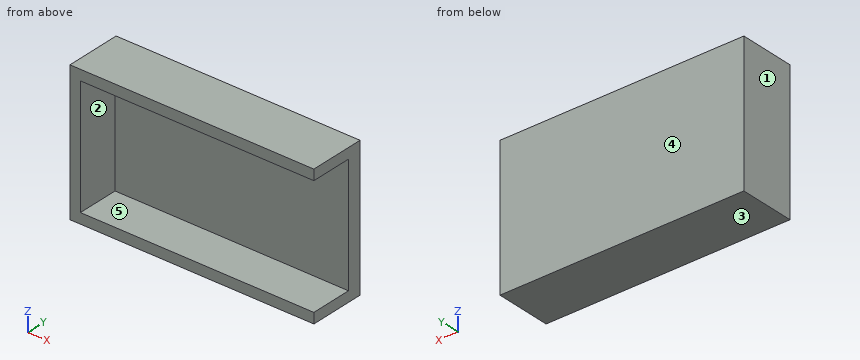
Autodesk Inventor part; units mm, degrees
ref_plane "YZ Plane" through (0, 0, 0) normal (1, 0, 0) x (0, 1, 0)
ref_plane "XZ Plane" through (0, 0, 0) normal (0, 1, 0) x (-1, 0, 0)
ref_plane "XY Plane" through (0, 0, 0) normal (0, 0, 1) x (1, 0, 0)
sketch "Эскиз1" plane through (0, 0, 0) normal (0, 1, 0) x (-1, 0, 0)
  line L0 (-35, 20) -> (35, 20)
  line L1 (35, 20) -> (35, -20)
  line L2 (35, -20) -> (-35, -20)
  line L3 (-35, -20) -> (-35, 20)
  line L4 (-35, 20) -> (35, -20) construction
  line L5 (35, 20) -> (-35, -20) construction
  point P0 (0, 0)
  dimension "d0" = 40
  dimension "d1" = 70
extrude "Выдавливание1" add sketch "Эскиз1" along normal blind 4
sketch "Эскиз2" plane through (0, 0, 0) normal (0, -1, 0) x (1, 0, 0)
  line L0 (-35, 20) -> (35, 20)
  line L1 (35, 20) -> (-35, 20)
  line L2 (-35, 20) -> (-35, 17)
  line L3 (-35, 17) -> (35, 17)
  line L4 (35, 17) -> (35, 20)
  line L5 (35, -20) -> (-35, -20)
  line L6 (35, -20) -> (-35, -20)
  line L7 (-35, -20) -> (-35, -17)
  line L8 (-35, -17) -> (35, -17)
  line L9 (35, -17) -> (35, -20)
  line L10 (-35, -20) -> (-35, 20)
  line L11 (-35, 17) -> (-32, 17)
  line L12 (-32, 17) -> (-32, -17)
  line L13 (-32, -17) -> (-35, -17)
  line L14 (-35, -17) -> (-35, 17)
  point P0 (0, 0)
  dimension "d4" = 3
extrude "Выдавливание2" add sketch "Эскиз2" along normal blind 12
properties part number "Battery box under the board"
Build history of the part. All positions in model axes, mm. Face numbers are marked on the shaded views. A direction names the side the tool comes from. Give positions to 0.01 mm unless a question says otherwise; leave off trailing zeros. Order: outer loops, then holes, each group sorted by start corner. A loop starts at its lowest first (then second) coordinate and runs counter-clockwise, first axis right, second up. Notation, with made-up numbers: M 63.25,33 L 94.25,33 A22 cw 94.25,58 Z; hole C 34.25,-4 d3. An arc over 180 degrees is marked long. Return JSON: item names as keys, results as strings.
Q1. Two-plate mould, pull along Z, no slides. Class the marked faces 3, 4 and 5: pulls with the +Z half, pulls with the -Z half, needs draft (parallel to the pull), parting line crosses it, or undercut.
Answer list:
{"face 3": "pulls with the -Z half", "face 4": "needs draft", "face 5": "undercut"}
Q2. Band-saw the part on A-A (y = -2.25). Give the cut face in (x, z), then the cut area to 3 significant figures.
Answer list:
{"outline": "M -35,-20 L 35,-20 L 35,-17 L -32,-17 L -32,17 L 35,17 L 35,20 L -35,20 Z", "area": "522 mm^2"}
Q3. Wall check: probe 1 along Z at (x, y) = (-15, -4.5); probe 2 along Y at (x, z) = (-18.5, 3); probe 3 along X at (y, z) = (-11, 3). Give the ranges that are in metal, low to high. Write a range as from..to.
Answer list:
{"probe 1": "z = -20..-17, 17..20", "probe 2": "y = 0..4", "probe 3": "x = -35..-32"}
Q4. Flat gauge pins, fed straight in: pin 1 (2 mm diameter, centred on x = -6, z = -7, fed in from -Y); pin 2 (5 mm diameter, centred on y = -7, z = -11.5, fed in from +X); pin 3 (4 mm diameter, centred on x = 1, z = -15.5, fed in from -Y). Where does each tip first touch, or does it go through?
Answer list:
{"pin 1": "stops at y = 0", "pin 2": "stops at x = -32", "pin 3": "stops at y = -12"}
Q5. Band-saw the part on B-B (z = 11.5). Give the cut face in (x, y), then the cut area to 3 significant figures.
Answer list:
{"outline": "M -35,-12 L -32,-12 L -32,0 L 35,0 L 35,4 L -35,4 Z", "area": "316 mm^2"}
Q6. Band-saw the part on C-C (x = -7). Give the cut face in (y, z), then the cut area to 3 significant figures.
Answer list:
{"outline": "M -12,-20 L 4,-20 L 4,20 L -12,20 L -12,17 L 0,17 L 0,-17 L -12,-17 Z", "area": "232 mm^2"}
Q7. 3-axis set-ups, long thin cutter, end or side, ignore diameter. For the marked faces 1 and 2: which of +Z, -Z, +X, -X, +Y, -Y reach the whole face in a straight line?
Answer list:
{"face 1": "+Z, -Z, -X, +Y, -Y", "face 2": "+X, -Y"}
